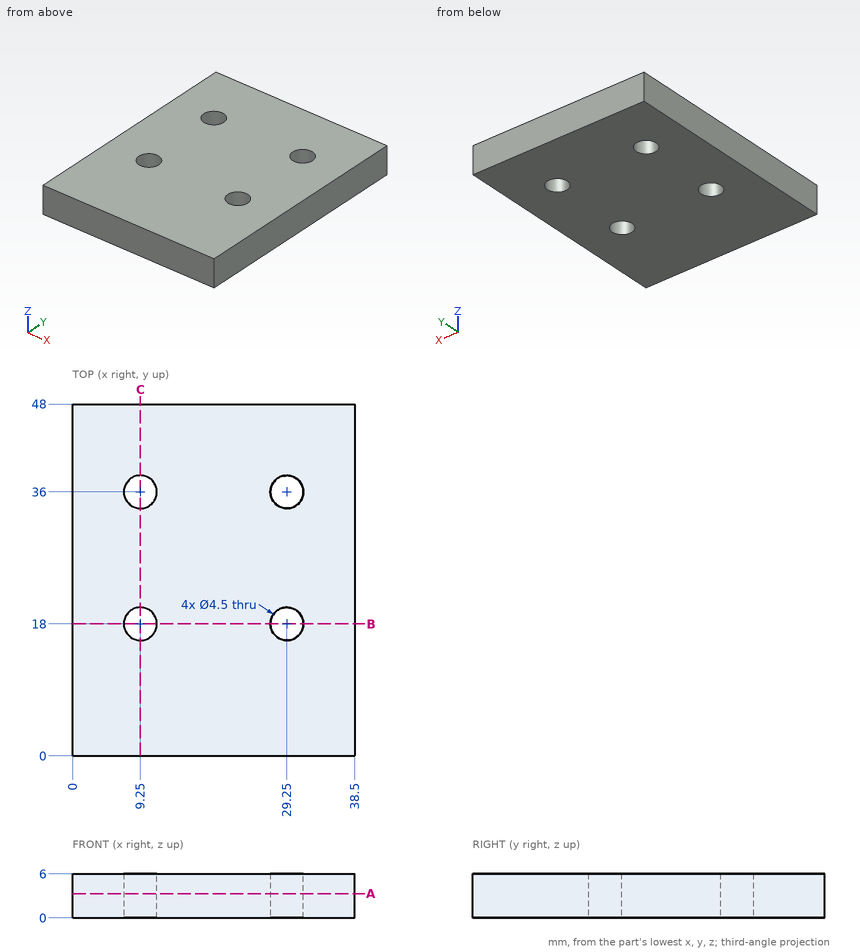
The figure shows three views and two pictorial views of one solid part (mm, origin at its lowest corner). Answer the questions. Round coordinates to 2 decimals unless told otherwise and drop trailing zeros. Write each loop counter-clockwise with the first axis right and the second up, starting at its lowest first coordinate (ties: lowest second). Pieces come first, ordered by that corner, then holes. Notation, with made-up numbers: (65.25, -35.75) - (81.25, -35.75) arc R16 ccw to (81.25, -5.75) - close; hole circle Ø6 at (42, 16). An arc over 180 degrees is marked (long way). One line per question, with ' | ' between items. Start each with the question number.
1. Section B-B (y = 18) is taken. Determine the outline of the cut face in (x, z).
2. Section C-C (x = 9.25) is taken. Determine the outline of the cut face in (y, z).
3. Section A-A (z = 3.3) is taken. Determine the outline of the cut face in (x, y), and give its area (3 significant figures).
4. Find the intervals of material crossed by probe 1 along Y at (x, z) = (29.25, 3.8); probe 2 along Y at (x, z) = (11, 2.8); probe 3 along X at (y, z) = (35.5, 3.75), in increasing order. Write a range as [from, to].
5. This flat-tipped pin is pushed along its axis until it touches: pin 1 (4 mm diameter, centred on x = 29.25, y = 36, fed in from +Z). Where does it stop, or does it pass through?
Filled in:
1) outline: (0, 0) - (7, 0) - (7, 6) - (0, 6) - close; (11.5, 0) - (27, 0) - (27, 6) - (11.5, 6) - close; (31.5, 0) - (38.5, 0) - (38.5, 6) - (31.5, 6) - close
2) outline: (0, 0) - (15.75, 0) - (15.75, 6) - (0, 6) - close; (20.25, 0) - (33.75, 0) - (33.75, 6) - (20.25, 6) - close; (38.25, 0) - (48, 0) - (48, 6) - (38.25, 6) - close
3) outline: (0, 0) - (38.5, 0) - (38.5, 48) - (0, 48) - close; hole circle Ø4.5 at (9.25, 18); hole circle Ø4.5 at (9.25, 36); hole circle Ø4.5 at (29.25, 18); hole circle Ø4.5 at (29.25, 36) | area: 1,780 mm²
4) probe 1: [0, 15.75], [20.25, 33.75], [38.25, 48] | probe 2: [0, 16.59], [19.41, 34.59], [37.41, 48] | probe 3: [0, 7.06], [11.44, 27.06], [31.44, 38.5]
5) pin 1: through
